```python
from build123d import *

# Parameters (mm, degrees)
SKETCH1_W               = 26
SKETCH1_H               = 43.24
BOSS_EXTRUDE1_DEPTH     = 16
CUT_EXTRUDE1_DEPTH      = 39.06079873
CUT_EXTRUDE1_DEPTH_BACK = 39.06079873
SKETCH2_R               = 0.55
SKETCH2_R_2             = 1.7
SKETCH3_W               = 14.5
SKETCH3_H               = 20.24
CUT_EXTRUDE3_DEPTH      = 4
SKETCH4_R               = 1
CUT_EXTRUDE5_DEPTH      = 10


with BuildPart() as part:
    # Sketch1 → Boss-Extrude1 (new body)
    with BuildSketch(Plane.XY):
        with Locations((9, 5)):
            Rectangle(SKETCH1_W, SKETCH1_H)
    extrude(amount=BOSS_EXTRUDE1_DEPTH)

    # Sketch2 → Cut-Extrude1 (cut, two sides: drawn at the far end of the back side and taken through both)
    with BuildSketch(Plane.XY.offset(-CUT_EXTRUDE1_DEPTH_BACK)):
        with Locations((8, -2.62)):
            Circle(SKETCH2_R)
        with Locations((8, 2.46)):
            Circle(SKETCH2_R)
        with Locations((8, 7.54)):
            Circle(SKETCH2_R)
        with Locations((8, 12.62)):
            Circle(SKETCH2_R)
        with Locations((8, -12.87)):
            Circle(SKETCH2_R_2)
        with Locations((8, 22.87)):
            Circle(SKETCH2_R_2)
    extrude(amount=CUT_EXTRUDE1_DEPTH + CUT_EXTRUDE1_DEPTH_BACK, mode=Mode.SUBTRACT)

    # Sketch3 → Cut-Extrude3 (cut)
    with BuildSketch(Plane.XY):
        with Locations((3.25, 5)):
            Rectangle(SKETCH3_W, SKETCH3_H)
    extrude(amount=CUT_EXTRUDE3_DEPTH, mode=Mode.SUBTRACT)

    # Sketch4 → Cut-Extrude5 (cut)
    with BuildSketch(Plane.XY.offset(16)):
        with Locations((8, -6.62)):
            Circle(SKETCH4_R)
        with Locations((8, 16.62)):
            Circle(SKETCH4_R)
    extrude(amount=-CUT_EXTRUDE5_DEPTH, mode=Mode.SUBTRACT)


solid = part.part
```
Design review of the part built by this model. Coordinates are the model's own, in mm. A direction names the side the tool comes from. Round coordinates to 2 decimals unless told otherwise and drop trailing zeros. Write each loop counter-clockwise with the first axis right and the second up, starting at its lowest first coordinate (ties: lowest second). Pieces come first, ordered by that corner, then holes. Notation, with made-up numbers: (-1.5, 52) -> (47.5, 52) arc R15 ccw to (47.5, 76) -> close; hole circle Ø6 at (52.5, 15). An arc over 180 degrees is marked (long way). Write item = value, one per line. Start each with the question number.
1) Take a section at B-B, the plane y = -12.87. State the section outline as (x, z) points.
2) Wall thickness on probe 1 along X at (y, z) = (-6.5, 14); probe 2 along X at (y, z) = (-2.62, 8); probe 3 along Z at (x, y) = (1.25, 4): over which ranges is each line inside the solid? List them lowest first. Write a range as from..to.
3) Take a section at A-A, the plane z = 9. Count the separate pieces of the cut face and the enclosed holes in it, plus the area to 3 significant figures.
4) Clearance check with flat-ended pins moving along their axes: pin 1 (1.2 mm diameter, centred on y = 9, z = 1.5, fed in from -X); pin 2 (7 mm diameter, centred on x = 6, y = 7, fed in from -Z). State where each tip first meets the part, or that it passes through.
5) Take a section at C-C, the plane x = -0.75. State the section outline as (y, z) points.
6) Mouldability with a two-part tool opening along Y and no side actions: class faces 1 (the face through (-4, 5, 8)), 2 (the face through (9, 26.62, 8)), 3 (the face through (7.56, 12.29, 9.92)) as +Y half, -Y half, draft (parallel to the pull), parting line (faces both ways), or undercut.
7) Take a section at D-D, the plane y = 9.5. State the section outline as (x, z) points, plus the area to 3 significant figures.
8) Tool access review of faces 4 (the face through (9, 5, 16)), 5 (the face through (8, 17, 6)), 6 (the face through (3, 15.12, 2)): name each direction out of +Z, -Z, +X, -X, +Y, -Y from which nothing blocks a thin tool from reaching the whole face with its end or side.
Results list:
q1.outline = (-4, 0) -> (6.3, 0) -> (6.3, 16) -> (-4, 16) -> close; (9.7, 0) -> (22, 0) -> (22, 16) -> (9.7, 16) -> close
q2.probe_1 = -4..7.01, 8.99..22
q2.probe_2 = -4..7.45, 8.55..22
q2.probe_3 = 4..16
q3.separate_pieces = 1
q3.enclosed_holes = 8
q3.area = 1,100 mm²
q4.pin_1 = 10.5
q4.pin_2 = 4
q5.outline = (-16.62, 0) -> (-5.12, 0) -> (-5.12, 4) -> (15.12, 4) -> (15.12, 0) -> (26.62, 0) -> (26.62, 16) -> (-16.62, 16) -> close
q6.face_1 = draft
q6.face_2 = +Y half
q6.face_3 = undercut
q7.outline = (-4, 4) -> (10.5, 4) -> (10.5, 0) -> (22, 0) -> (22, 16) -> (-4, 16) -> close
q7.area = 358 mm²
q8.face_4 = +Z, +X, -X, +Y, -Y
q8.face_5 = +Z
q8.face_6 = -Z, -X
